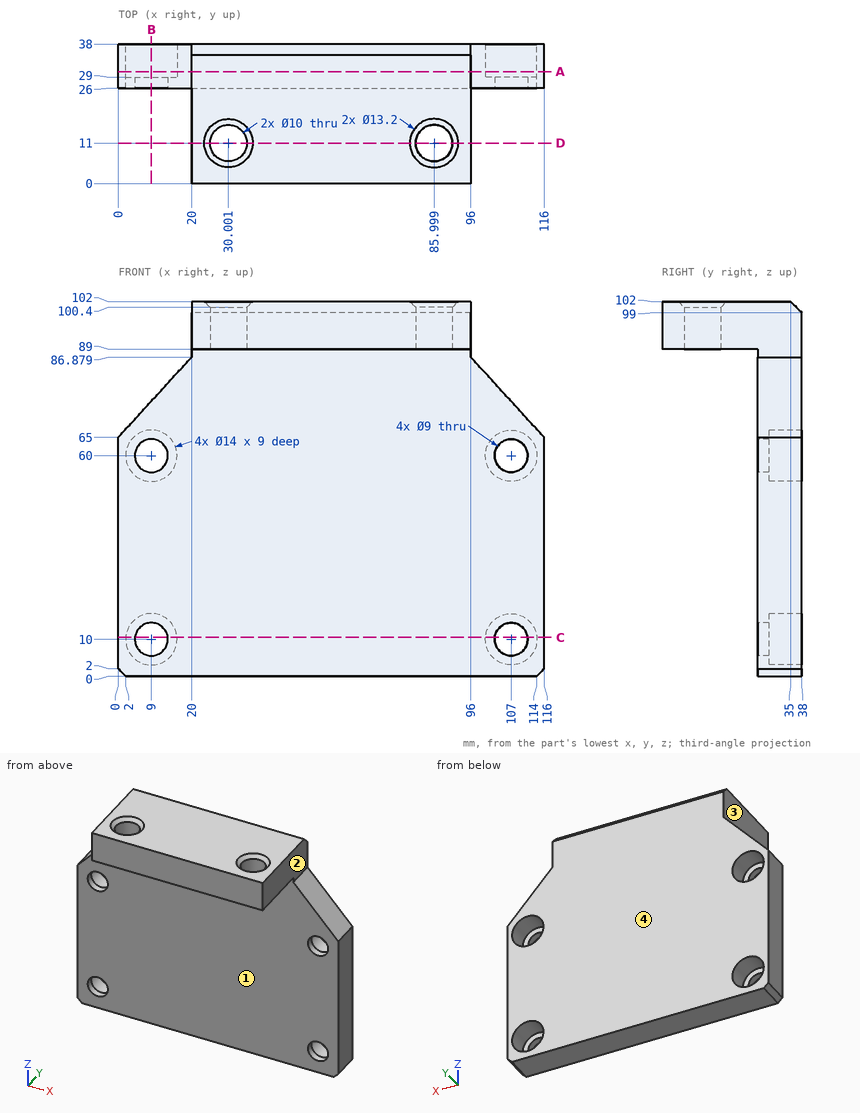
Geometry: see drawing. Coordinates: mm, zero at the bounding-box minimum. A direction names the side the tool comes from. Give positions to 0.01 mm unless a question says otherwise; leave off trailing zeros. Loops run counter-clockwise (first coordinate to the right, second up) from the corner with the lowest first, then second, coordinate; pieces in that order, holes last. Notation, with made-up numbers: (20.5, 72.5) -> (55.5, 72.5) arc R13 ccw to (55.5, 97.5) -> close; hole circle Ø9 at (83.25, -3.75). An arc over 180 degrees is marked (long way). Use CSV: the item, a comma, the result in double quotes.
(1) Cut plane C-C (z = 10.5). Output: boundary loops of the cut face in (x, y).
From the geometry:
outline,"(0, 26) -> (4.53, 26) -> (4.53, 29) -> (2.02, 29) -> (2.02, 38) -> (0, 38) -> close; (13.47, 26) -> (102.53, 26) -> (102.53, 29) -> (100.02, 29) -> (100.02, 38) -> (15.98, 38) -> (15.98, 29) -> (13.47, 29) -> close; (111.47, 26) -> (116, 26) -> (116, 38) -> (113.98, 38) -> (113.98, 29) -> (111.47, 29) -> close"
(2) Cut plane B-B (x = 9). Output: boundary loops of the cut face in (y, z) (1 decimal).
From the geometry:
outline,"(26, 0) -> (38, 0) -> (38, 3) -> (29, 3) -> (29, 5.5) -> (26, 5.5) -> close; (26, 14.5) -> (29, 14.5) -> (29, 17) -> (38, 17) -> (38, 53) -> (29, 53) -> (29, 55.5) -> (26, 55.5) -> close; (26, 64.5) -> (29, 64.5) -> (29, 67) -> (38, 67) -> (38, 74.8) -> (26, 74.8) -> close"
(3) Cut plane A-A (y = 30.5). Output: boundary loops of the cut face in (x, z).
From the geometry:
outline,"(0, 2) -> (2, 0) -> (114, 0) -> (116, 2) -> (116, 65) -> (96, 86.88) -> (96, 102) -> (20, 102) -> (20, 86.88) -> (0, 65) -> close; hole circle Ø14 at (9, 10); hole circle Ø14 at (9, 60); hole circle Ø14 at (107, 10); hole circle Ø14 at (107, 60)"
(4) First-contact query: P1, Ø9, axis at x = 86, y = 11, coming from the +Z side; P2, Ø16.5, axis at y = 27, z = 92.5, coming from the +X side; P3, Ø12.5, axis at x = 107, z = 60, coming from the +Y side; P4, Ø16.5, axis at y = 15.5, z = 94.5, coming from the -X side. Flat tips, straight axial feed; report the tip coordinate or a pass-through.
From the geometry:
P1,"through"
P2,"x = 98.4"
P3,"y = 29"
P4,"x = 20"
(5) Cut plane D-D (y = 11). Output: boundary loops of the cut face in (x, z), plus the area to 3 significant figures.
From the geometry:
outline,"(20, 89) -> (25, 89) -> (25, 100.4) -> (23.4, 102) -> (20, 102) -> close; (35, 89) -> (81, 89) -> (81, 100.4) -> (79.4, 102) -> (36.6, 102) -> (35, 100.4) -> close; (91, 89) -> (96, 89) -> (96, 102) -> (92.6, 102) -> (91, 100.4) -> close"
area,"723 mm^2"
(6) Ray query, line 1 along X through (y, z) = (34.75, 10); line 2 along Z through (x, y) = (9, 31) (1 decimal); line 3 along X through (y, z) = (35.5, 4) (1 decimal). Return the intervals inside material, ascending. Write a range as [from, to].
From the geometry:
line 1,"[0, 2], [16, 100], [114, 116]"
line 2,"[0, 3], [17, 53], [67, 74.8]"
line 3,"[0, 5.4], [12.6, 103.4], [110.6, 116]"
(7) Access query for the marked faces 1, 2, 3 and 4. Directions: +Z, -Z, +X, -X, +Y, -Y. A direction counts if a zero-diameter tool reaches every point of the face in a straight line with its end or side. Return the directions, or none.
From the geometry:
face 1,"-Z, +X, -X, -Y"
face 2,"+Z, +X, +Y, -Y"
face 3,"+Z, -X, +Y, -Y"
face 4,"+Z, -Z, +X, -X, +Y"
